from build123d import *

# Parameters (mm, degrees)
SKETCH005_W     = 42
SKETCH005_H     = 42
PAD004_DEPTH    = 22.75
CHAMFER001_SIZE = 7.5
SKETCH008_R     = 1.22
POCKET001_DEPTH = 22.751
SKETCH012_R     = 18
POCKET006_DEPTH = 22.751


with BuildPart() as part:
    # Sketch005 → Pad004 (new body)
    with BuildSketch(Plane.XY):
        Rectangle(SKETCH005_W, SKETCH005_H)
    extrude(amount=PAD004_DEPTH)

    # Chamfer001
    chamfer001_edges = [part.edges().sort_by_distance(p)[0] for p in [
        (-21, -21, 11.375),
        (-21, 21, 11.375),
        (21, -21, 11.375),
        (21, 21, 11.375),
    ]]
    chamfer(chamfer001_edges, length=CHAMFER001_SIZE)

    # Sketch008 (on Face2 of Chamfer001) → Pocket001 (cut, through all)
    with BuildSketch(Plane(origin=(0, 0, 0), x_dir=(1, 0, 0), z_dir=(0, 0, -1))):
        with Locations((-15.5, 15.5)):
            Circle(SKETCH008_R)
        with Locations((15.5, 15.5)):
            Circle(SKETCH008_R)
        with Locations((15.5, -15.5)):
            Circle(SKETCH008_R)
        with Locations((-15.5, -15.5)):
            Circle(SKETCH008_R)
    extrude(amount=-POCKET001_DEPTH, mode=Mode.SUBTRACT)

    # Sketch012 (on Face5 of Pocket001) → Pocket006 (cut, through all)
    with BuildSketch(Plane.XY.offset(22.75)):
        Circle(SKETCH012_R)
    extrude(amount=-POCKET006_DEPTH, mode=Mode.SUBTRACT)


with BuildPart() as part_1:
    # Body003 placement: moved
    add(part.part.moved(Location((0, 0, 9.6))))


solid = part_1.part
The model under review builds one solid part; all positions refer to its coordinate system, in mm. Give positions to 0.01 mm unless a question says otherwise; leave off trailing zeros. Loops run counter-clockwise (first coordinate to the right, second up) from the corner with the lowest first, then second, coordinate; pieces in that order, holes last. Notation, with made-up numbers: (15.25, 52.25) -> (38.25, 52.25) arc R19 cw to (38.25, 78.25) -> close; hole circle Ø6 at (-34.5, 76.25). An arc over 180 degrees is marked (long way). Put each result on its own line as item: value. Start each with the question number.
1. We need section B-B on y = 0. State the section outline as (x, z) points, then the cut area to 4 significant figures.
2. Clearance check with a flat-ended pin moving along its axis: P1, Ø1.5, axis at x = -15.5, y = 15.5, coming from the -Z side. State where the tip first meets the part, or that it passes through.
3. Wall thickness on probe 1 along Y at (x, z) = (0, 16.25); probe 2 along Y at (x, z) = (16, 22.5); probe 3 along X at (y, z) = (-15.5, 23.25): over which ranges is each line inside the solid? List them lowest first.
4. We need section D-D on y = 15.5. State the section outline as (x, z) points.
5. We need section A-A on z = 14.5. State the section outline as (x, y) points.
6. Mouldability with a two-part tool opening along Y and no side actions: class faces 1 (the face through (-14.8, -16.5, 20.8)), 2 (the face through (17.3, -17.2, 20.8)), 3 (the face through (-2.343, 17.847, 21.134)), 4 (the face through (17.2, 17.3, 20.8)) as released by +Y, released by -Y, zero draft, split by the parting line, or undercut.
Determined:
1. outline: (-21, 9.6) -> (-18, 9.6) -> (-18, 32.35) -> (-21, 32.35) -> close; (18, 9.6) -> (21, 9.6) -> (21, 32.35) -> (18, 32.35) -> close
1. area: 136.5 mm^2
2. P1: through
3. probe 1: -21 to -18, 18 to 21
3. probe 2: -18.5 to -16.61, -14.39 to -8.25, 8.25 to 14.39, 16.61 to 18.5
3. probe 3: -19 to -16.72, -14.28 to -9.15, 9.15 to 14.28, 16.72 to 19
4. outline: (-19, 9.6) -> (-16.72, 9.6) -> (-16.72, 32.35) -> (-19, 32.35) -> close; (-14.28, 9.6) -> (-9.15, 9.6) -> (-9.15, 32.35) -> (-14.28, 32.35) -> close; (9.15, 9.6) -> (14.28, 9.6) -> (14.28, 32.35) -> (9.15, 32.35) -> close; (16.72, 9.6) -> (19, 9.6) -> (19, 32.35) -> (16.72, 32.35) -> close
5. outline: (-21, -13.5) -> (-13.5, -21) -> (13.5, -21) -> (21, -13.5) -> (21, 13.5) -> (13.5, 21) -> (-13.5, 21) -> (-21, 13.5) -> close; hole circle Ø36 at (0, 0); hole circle Ø2.44 at (-15.5, -15.5); hole circle Ø2.44 at (-15.5, 15.5); hole circle Ø2.44 at (15.5, -15.5); hole circle Ø2.44 at (15.5, 15.5)
6. face 1: undercut
6. face 2: released by -Y
6. face 3: undercut
6. face 4: released by +Y
